Design review of the part built by this model. Coordinates are the model's own, in mm. A direction names the side the tool comes from. Coordinates: 2 decimals unless noted, no trailing zeros. Order: outer loops, then holes, each group sorted by start corner. A loop starts at its lowest first (then second) coordinate and runs counter-clockwise, first axis right, second up. Notation, with made-up numbers: (12.5, -6.5) -> (48.5, -6.5) arc R21 ccw to (48.5, 6.5) -> close; hole circle Ø3 at (75.5, -13). An arc over 180 degrees is marked (long way). Write item = value, one per line.
```python
from build123d import *

# Parameters (mm, degrees)
SKETCH5_W       = 40
SKETCH5_H       = 17.5
EXTRUDE8_DEPTH  = 6
SKETCH7_R       = 5
EXTRUDE9_DEPTH  = 3
SKETCH8_R       = 4
EXTRUDE10_DEPTH = 3


with BuildPart() as part:
    # Sketch5 → Extrude8 (new body)
    with BuildSketch(Plane(origin=(0, 0, 0), x_dir=(1, 0, 0), z_dir=(0, 1, 0))):
        Rectangle(SKETCH5_W, SKETCH5_H)
    extrude(amount=EXTRUDE8_DEPTH)

    # Sketch7 → Extrude9 (cut)
    with BuildSketch(Plane.XZ):
        with Locations(Location((-10, 0, 0), (0, 0, 270))):  # turned: the seam where the file's is
            Circle(SKETCH7_R)
    extrude9 = extrude(amount=-EXTRUDE9_DEPTH, mode=Mode.SUBTRACT)

    # Sketch8 → Extrude10 (cut)
    with BuildSketch(Plane.XZ.offset(-3)):
        with Locations(Location((-10, 0, 0), (0, 0, 270))):  # turned: the seam where the file's is
            Circle(SKETCH8_R)
    extrude10 = extrude(amount=-EXTRUDE10_DEPTH, mode=Mode.SUBTRACT)

    # Mirror2: Extrude9, Extrude10 across plane
    add(extrude9.mirror(Plane(origin=(0, 0, 0), x_dir=(0, 0, 1), z_dir=(1, 0, 0))), mode=Mode.SUBTRACT)
    add(extrude10.mirror(Plane(origin=(0, 0, 0), x_dir=(0, 0, 1), z_dir=(1, 0, 0))), mode=Mode.SUBTRACT)


solid = part.part
```
(1) The part is to be moulded in two halves that separate along X. For faces 1 (the flat face through (0, 0, 0)), 2 (the flat face through (-20, 3, 0)), 3 (the cylindrical face through (-6, 1, -3)), say which applies: released by +X, released by -X, zero draft, split by the parting line, or undercut.
Report:
face_1 = zero draft
face_2 = released by -X
face_3 = undercut
(2) For faces 4 (the cylindrical face through (6, 1, -3)), 5 (the cylindrical face through (-13.905, 4.479, 0.867)), list the 3-axis set-ups (+Z, -Z, +X, -X, +Y, -Y) from which the entire face can be reached by the end or side of a thin tool; tool diameter is ignored.
Report:
face_4 = -Y
face_5 = +Y, -Y
(3) We need section C-C (y = 2.4). Write out the cut boundary in (x, z), and give its area (3 significant figures).
Report:
outline = (-20, -8.75) -> (20, -8.75) -> (20, 8.75) -> (-20, 8.75) -> close; hole circle Ø10 at (-10, 0); hole circle Ø10 at (10, 0)
area = 543 mm²
(4) For L1, parallel to X at y = 4.6, z = 0; L2, parallel to X at y = 1, z = 0; L3, parallel to Z at x = 10, y = 4.7, list the stretches that pass through material, from the lowest coordinate up.
Report:
L1 = -20 to -14, -6 to 6, 14 to 20
L2 = -20 to -15, -5 to 5, 15 to 20
L3 = -8.75 to -4, 4 to 8.75
(5) We need section B-B (x = 10). Write out the cut boundary in (y, z), and give its area (3 significant figures).
Report:
outline = (0, -8.75) -> (6, -8.75) -> (6, -4) -> (3, -4) -> (3, -5) -> (0, -5) -> close; (0, 5) -> (3, 5) -> (3, 4) -> (6, 4) -> (6, 8.75) -> (0, 8.75) -> close
area = 51.0 mm²
(6) We need section A-A (z = 0). Write out the cut boundary in (x, y), and give its area (3 significant figures).
Report:
outline = (-20, 0) -> (-15, 0) -> (-15, 3) -> (-14, 3) -> (-14, 6) -> (-20, 6) -> close; (-6, 3) -> (-5, 3) -> (-5, 0) -> (5, 0) -> (5, 3) -> (6, 3) -> (6, 6) -> (-6, 6) -> close; (14, 3) -> (15, 3) -> (15, 0) -> (20, 0) -> (20, 6) -> (14, 6) -> close
area = 132 mm²
(7) We need section D-D (z = 4.5). Write out the cut boundary in (x, y).
Report:
outline = (-20, 0) -> (-12.18, 0) -> (-12.18, 3) -> (-7.82, 3) -> (-7.82, 0) -> (7.82, 0) -> (7.82, 3) -> (12.18, 3) -> (12.18, 0) -> (20, 0) -> (20, 6) -> (-20, 6) -> close
